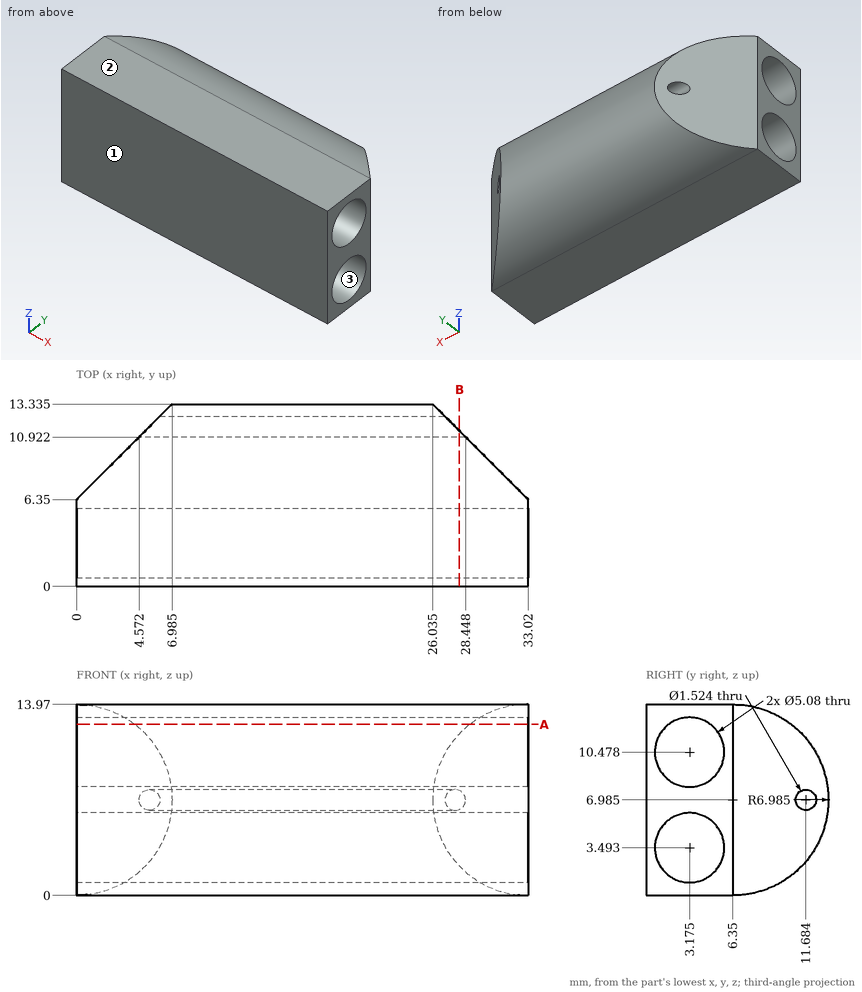
Answer from the drawing. Dimensions are ordinates in mm from the lowest x, y and z of the part. Coordinates: 2 decimals unless noted, no trailing zeros. Loops run counter-clockwise (first coordinate to the right, second up) from the corner with the lowest first, then second, coordinate; pieces in that order, holes last.
Q1. Each of these flat-tipped pins is pushed along its axis until it touches: pin 1 Ø5 at (x, y) = (25.5, 11.5) entering from -Z; pin 2 Ø4 at (y, z) = (3.18, 10.48) entering from -X. Where does it stop, or does it pass through?
Q2. The part is cut by section B-B on x = 28. Give the number of separate pieces and of enclosed holes in the cut face, and give its area (3 significant figures).
Q3. Consider probe 1 along Z at (x, y) = (4, 3.25); probe 2 along Z at (x, y) = (28, 5) (1 decimal); probe 3 along Z at (x, y) = (27, 12) (1 decimal). Determine where each line is inside the solid, lowest interval first.
Q4. The mould has two halves that part along Y. Classify the marked faces 1, 2 and 3: +Y half, -Y half, draft (parallel to the pull), parting line (faces both ways), or undercut.
Q5. The part is cut by section A-A on z = 12.5. Write down the section's boundary in (x, y).
Results below:
1. pin 1: stops at z = 0.52
1. pin 2: passes through
2. separate pieces: 1
2. enclosed holes: 2
2. area: 111 mm2
3. probe 1: z = 0 to 0.95, 6.03 to 7.94, 13.02 to 13.97
3. probe 2: z = 0 to 1.7, 5.3 to 8.7, 12.2 to 14
3. probe 3: z = 2.9 to 6.3, 7.7 to 11.1
4. face 1: -Y half
4. face 2: draft
4. face 3: undercut
5. outline: (0, 0) - (33.02, 0) - (33.02, 1.64) - (0, 1.64) - close; (0, 4.71) - (33.02, 4.71) - (33.02, 6.35) - (28.73, 10.64) - (4.29, 10.64) - (0, 6.35) - close
